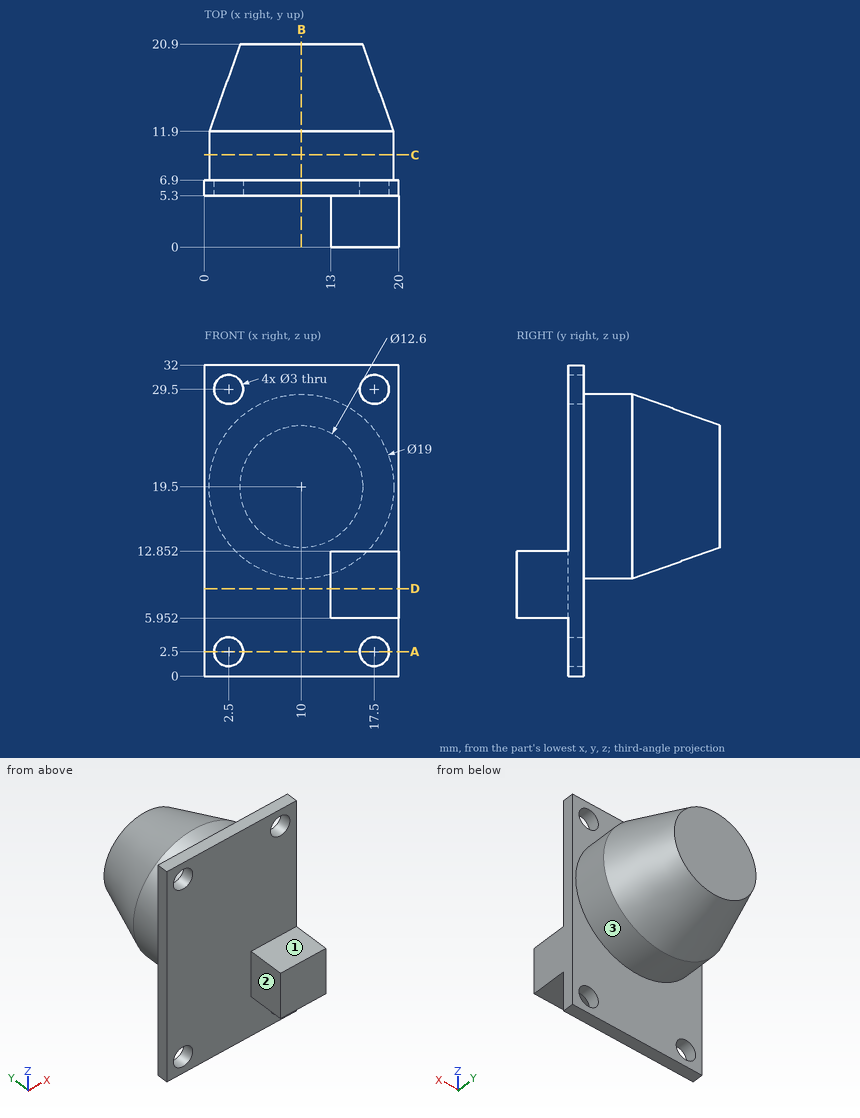
Could you check a few things on this drawing? It's one solid part, dimensions in mm from its lowest x, y, z. A direction names the side the tool comes from. Round coordinates to 2 decimals unless told otherwise and drop trailing zeros. Loops run counter-clockwise (first coordinate to the right, second up) from the corner with the lowest first, then second, coordinate; pieces in that order, holes last.
Q1. Please list where these lines run through material, in increasing order: L1, parallel to X at y = 5.9, z = 2.5; L2, parallel to Z at x = 2.5, y = 6.05; L3, parallel to Y at x = 18.5, z = 25.5.
Q2. I want a section at D-D (z = 9). Write out the boundary of the cut face in (x, y), and give its area (3 significant figures).
Q3. I want a section at B-B (x = 10). Write out the boundary of the cut face in (y, z), and give its area (3 significant figures).
Q4. I want a section at C-C (y = 9.5). Write out the boundary of the cut face in (x, z), and give its area (3 significant figures).
Q5. On a 3-axis mill with a long thin cutter (end or side, diameter ignored), from which of +Z, -Z, +X, -X, +Y, -Y can I reach the whole of each face in a straight line? I mean the marked faces 1, 2 and 3. Say none if no direction works.
Q6. I want a section at A-A (z = 2.5). Write out the boundary of the cut face in (x, y).
Q7. For P1, Ø1.5, axis at x = 9, z = 22, coming from the -Y side; P2, Ø4, axis at x = 17.5, y = 9.5, coming from the +Z side; P3, Ø3, axis at x = 4.5, y = 14, coming from the -Z side, each with a flat end and sliding along its axis, tell me the tip position at first contact or that it passes through.
Answer below:
1. L1: x = 0 to 1, 4 to 16, 19 to 20
1. L2: z = 0 to 1, 4 to 28, 31 to 32
1. L3: y = 5.3 to 6.9
2. outline: (0, 5.3) - (13, 5.3) - (13, 0) - (20, 0) - (20, 6.9) - (0, 6.9) - close
2. area: 69.1 mm2
3. outline: (5.3, 0) - (6.9, 0) - (6.9, 10) - (11.9, 10) - (20.9, 13.2) - (20.9, 25.8) - (11.9, 29) - (6.9, 29) - (6.9, 32) - (5.3, 32) - close
3. area: 288 mm2
4. outline: circle Ø19 at (10, 19.5)
4. area: 284 mm2
5. face 1: +Z, +X, -X, -Y
5. face 2: +Z, -Z, -X, -Y
5. face 3: +Y
6. outline: (0, 5.3) - (1, 5.3) - (1, 6.9) - (0, 6.9) - close; (4, 5.3) - (16, 5.3) - (16, 6.9) - (4, 6.9) - close; (19, 5.3) - (20, 5.3) - (20, 6.9) - (19, 6.9) - close
7. P1: stops at y = 5.3
7. P2: stops at z = 27.25
7. P3: stops at z = 11.51
